Can you work these out from the model? Positions are in its coordinate system, mm. A direction names the side the tool comes from. Give positions to 0.01 mm unless a question says otherwise; leave off trailing zeros. Loops run counter-clockwise (first coordinate to the right, second up) from the corner with the lowest first, then second, coordinate; pieces in that order, holes last. Notation, with made-up numbers: (11.5, -30) -> (24.5, -30) arc R33 ccw to (24.5, 5) -> close; hole circle Ø10 at (28.25, 37). An arc over 180 degrees is marked (long way). Return JSON: item names as keys, results as strings. Group by question number.
Q1. Will these pins go through, and if not, where does the flat tip stop? pin 1 (2 mm diameter, centred on y = -43.5, z = 6.5, fed in from -X); pin 2 (1.2 mm diameter, centred on x = 33, z = 7, fed in from -Y); pin 3 (1 mm diameter, centred on x = 23, y = -46, fed in from +Z).
Q2. Which directions (+Z, -Z, +X, -X, +Y, -Y) give clear straight access to the entire face, cutting with the end or side of a thin tool? Please do faces 5 (the flat face through (36.5, -42, 7)), 6 (the flat face through (-34, 0, 0)), 7 (the cylindrical face through (38.4, -40.52, -4.93)).
Q3. I need wall thicknesses on line 1 along X through (y, z) = (-51, 2.25); line 2 along Z through (x, y) = (-24, -17); line 3 along X through (y, z) = (-58.5, 4.5). Which ranges of each line are inside material? Lowest first, please. Write a range as [from, to].
Q4. Suppose I cut it at C-C, the plane y = -45. Please give me the cut outline in (x, z).
Q5. Suppose I cut it at A-A, the plane x = -4. Please give me the cut outline in (y, z).
Q6. Suppose I cut it at B-B, the plane z = -0.75. Please give me the cut outline in (x, y), and give its area (3 significant figures).
Q7. Thinking about a two-plate mould opening in Z: for faces 1 (the cylindrical face through (42, -40.49, -6.57)), 2 (the flat face through (-0.2, -5, -3.3)), 3 (the flat face through (31.597, -3, 5)), 4 (the flat face through (37, -37, 8)), which applies, pulls with the +Z half, pulls with the -Z half, needs draft (parallel to the pull), parting line crosses it, or undercut?
```python
from build123d import *

# Parameters (mm, degrees)
F0_W     = 87
F0_H     = 16
F1_DEPTH = 75
F2_R     = 5
F3_W     = 78
F3_H     = 11
F4_DEPTH = 70
F5_W     = 73
F5_H     = 68
F6_DEPTH = 2.5
F7_R     = 2
F8_W     = 63.19318
F8_H     = 17.0015
F9_DEPTH = 25
F10_R    = 1


with BuildPart() as f1:
    # F0 (on Front) → F1 (new body)
    with BuildSketch(Plane.XZ):
        Rectangle(F0_W, F0_H)
    extrude(amount=F1_DEPTH)

    # F2
    f2_edges = [f1.edges().sort_by_distance(p)[0] for p in [
        (-43.5, -37.5, 8),
        (43.5, -37.5, 8),
        (43.5, -37.5, -8),
        (-43.5, -37.5, -8),
        (0, 0, 8),
        (0, 0, -8),
        (-43.5, 0, 0),
        (43.5, 0, 0),
    ]]
    fillet(f2_edges, radius=F2_R)

    # F3 (on face) → F4 (cut)
    with BuildSketch(Plane.XZ.offset(75)):
        Rectangle(F3_W, F3_H)
    extrude(amount=-F4_DEPTH, mode=Mode.SUBTRACT)

    # F5 (on face) → F6 (cut, through all)
    with BuildSketch(Plane.XY.offset(8)):
        with Locations((0, -41)):
            Rectangle(F5_W, F5_H)
    extrude(amount=-F6_DEPTH, mode=Mode.SUBTRACT)

    # F7
    f7_edges = [f1.edges().sort_by_distance(p)[0] for p in [
        (36.5, -7, 6.75),
        (-36.5, -7, 6.75),
        (39, -40, -5.5),
        (0, -5, -5.5),
        (-39, -40, -5.5),
        (-39, -5, 0),
        (39, -5, 0),
    ]]
    fillet(f7_edges, radius=F7_R)

    # F8 (on face) → F9 (cut)
    with BuildSketch(Plane(origin=(0, 0, 0), x_dir=(-1, 0, 0), z_dir=(0, 1, 0))):
        with BuildLine():
            ThreePointArc((-31.59659, 2), (-30.132124, -1.535534), (-26.59659, -3))
            Line((-26.59659, -3), (26.59659, -3))
            ThreePointArc((26.59659, -3), (30.132124, -1.535534), (31.59659, 2))
            Line((31.59659, 2), (31.59659, 3))
            Line((31.59659, 3), (-31.59659, 3))
            Line((-31.59659, 3), (-31.59659, 2))
        make_face()
        with Locations((0, 11.50075)):
            Rectangle(F8_W, F8_H)
    extrude(amount=-F9_DEPTH, mode=Mode.SUBTRACT)

    # F10
    f10_edges = [f1.edges().sort_by_distance(p)[0] for p in [
        (39, -41, 5.5),
        (-39, -41, 5.5),
    ]]
    fillet(f10_edges, radius=F10_R)


solid = f1.part
```
Ans:
{
 "1": {"pin 1": "stops at x = -42.83", "pin 2": "stops at y = -7", "pin 3": "stops at z = -5.5"},
 "2": {"face 5": "+Z, -Y", "face 6": "+Z, -Z, +X, -X, +Y", "face 7": "-Y"},
 "3": {"line 1": "x = [-43.5, -39], [39, 43.5]", "line 2": "z = [-8, -5.5]", "line 3": "x = [-43.27, -39], [39, 43.27]"},
 "4": {"outline": "(-43.5, -3) arc R5 ccw to (-38.5, -8) -> (38.5, -8) arc R5 ccw to (43.5, -3) -> (43.5, 3) arc R5 ccw to (38.5, 8) -> (36.5, 8) -> (36.5, 5.5) -> (38, 5.5) arc R1 cw to (39, 4.5) -> (39, -3.5) arc R2 cw to (37, -5.5) -> (-37, -5.5) arc R2 cw to (-39, -3.5) -> (-39, 4.5) arc R1 cw to (-38, 5.5) -> (-36.5, 5.5) -> (-36.5, 8) -> (-38.5, 8) arc R5 ccw to (-43.5, 3) -> close"},
 "5": {"outline": "(-75, -8) -> (-5, -8) arc R5 ccw to (0, -3) -> (-5, -3) -> (-5, -3.5) arc R2 cw to (-7, -5.5) -> (-75, -5.5) -> close"},
 "6": {"outline": "(-43.5, -75) -> (-39, -75) -> (-39, -7) arc R2 cw to (-37, -5) -> (-30.77, -5) -> (-30.77, 0) -> (-38.5, 0) arc R5 ccw to (-43.5, -5) -> close; (30.77, -5) -> (37, -5) arc R2 cw to (39, -7) -> (39, -75) -> (43.5, -75) -> (43.5, -5) arc R5 ccw to (38.5, 0) -> (30.77, 0) -> close", "area": "748 mm^2"},
 "7": {"face 1": "pulls with the -Z half", "face 2": "undercut", "face 3": "needs draft", "face 4": "pulls with the +Z half"}
}
